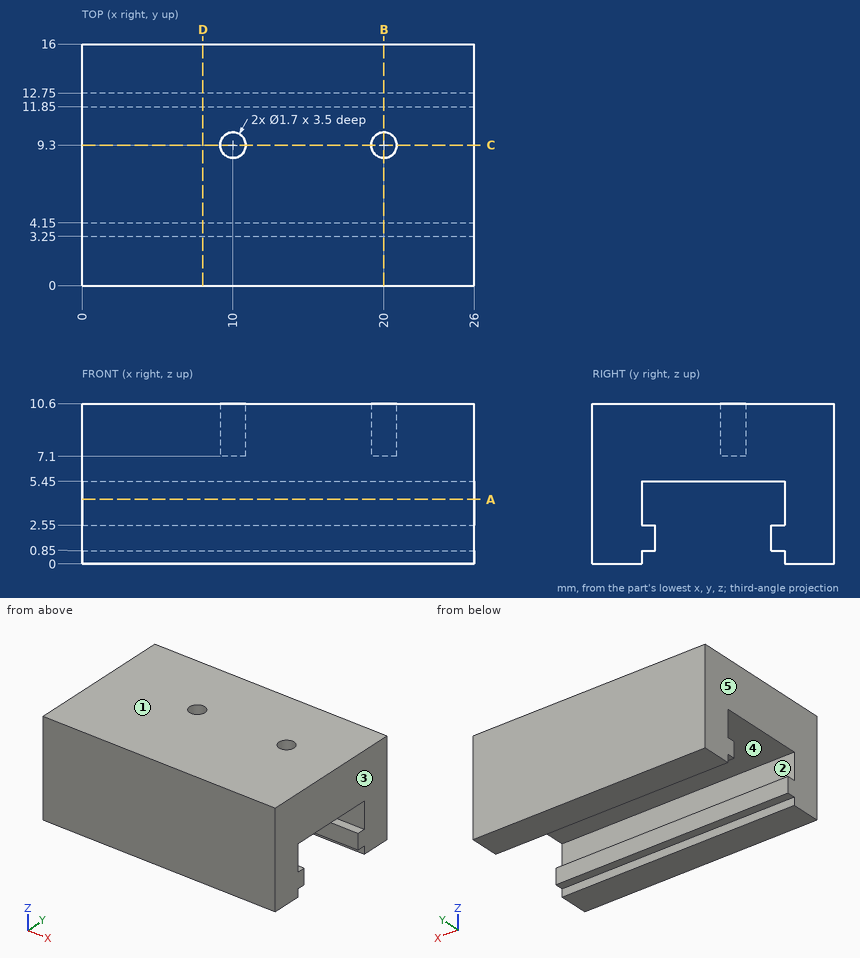
Answer from the drawing. Dimensions are ordinates in mm from the lowest x, y and z of the part. A direction names the side the tool comes from. Coordinates: 2 decimals unless noted, no trailing zeros. Order: outer loops, then holes, each group sorted by start corner. A loop starts at its lowest first (then second) coordinate and runs counter-clockwise, first axis right, second up. Notation, with made-up numbers: M 86.5,-38 L 144.5,-38 A31 ccw 144.5,1 Z; hole C 9,41.5 d11. An arc over 180 degrees is marked long. Put each result on its own line as item: value. Start each with the question number.
Item 1: Section B-B, the plane x = 20 is taken. Determine the outline of the cut face in (y, z).
Item 2: The mould has two halves that part along Z. Classify the marked faces 1, 2 and 3: +Z half, -Z half, draft (parallel to the pull), parting line (faces both ways), or undercut.
Item 3: Given pin 1 Ø1.5 at (x, y) = (20, 9.3) entering from -Z; pin 2 Ø0.5 at (x, y) = (20, 9) entering from +Z, each flat-ended and moving along its own axis, determine where each tip first touches the part or whether it passes through.
Item 4: Section A-A, the plane z = 4.25 is taken. Determine the outline of the cut face in (x, y).
Item 5: Consider probe 1 along X at (y, z) = (9.3, 9.55); probe 2 along Y at (x, z) = (24.75, 5.25); probe 3 along Z at (x, y) = (8.75, 12.25). Determine where each line is inside the solid, lowest interval first. Write a range as [from, to].
Item 6: For the marked faces 4 and 5, determine the directions among +Z, -Z, +X, -X, +Y, -Y from which every point of the face is accessible in a straight line to the end or side of a thin tool.
Item 7: Section D-D, the plane x = 8 is taken. Determine the outline of the cut face in (y, z), plus the area to 3 significant figures.
Item 8: Section C-C, the plane y = 9.3 is taken. Determine the outline of the cut face in (x, z).
Computed:
1. outline: M 0,0 L 3.25,0 L 3.25,0.85 L 4.15,0.85 L 4.15,2.55 L 3.25,2.55 L 3.25,5.45 L 12.75,5.45 L 12.75,2.55 L 11.85,2.55 L 11.85,0.85 L 12.75,0.85 L 12.75,0 L 16,0 L 16,10.6 L 10.15,10.6 L 10.15,7.1 L 8.45,7.1 L 8.45,10.6 L 0,10.6 Z
2. face 1: +Z half
2. face 2: undercut
2. face 3: draft
3. pin 1: stops at z = 5.45
3. pin 2: stops at z = 7.1
4. outline: M 0,0 L 26,0 L 26,3.25 L 0,3.25 Z; M 0,12.75 L 26,12.75 L 26,16 L 0,16 Z
5. probe 1: x = [0, 9.15], [10.85, 19.15], [20.85, 26]
5. probe 2: y = [0, 3.25], [12.75, 16]
5. probe 3: z = [0.85, 2.55], [5.45, 10.6]
6. face 4: +X, -X
6. face 5: +Z, -Z, -X, +Y, -Y
7. outline: M 0,0 L 3.25,0 L 3.25,0.85 L 4.15,0.85 L 4.15,2.55 L 3.25,2.55 L 3.25,5.45 L 12.75,5.45 L 12.75,2.55 L 11.85,2.55 L 11.85,0.85 L 12.75,0.85 L 12.75,0 L 16,0 L 16,10.6 L 0,10.6 Z
7. area: 121 mm2
8. outline: M 0,5.45 L 26,5.45 L 26,10.6 L 20.85,10.6 L 20.85,7.1 L 19.15,7.1 L 19.15,10.6 L 10.85,10.6 L 10.85,7.1 L 9.15,7.1 L 9.15,10.6 L 0,10.6 Z
